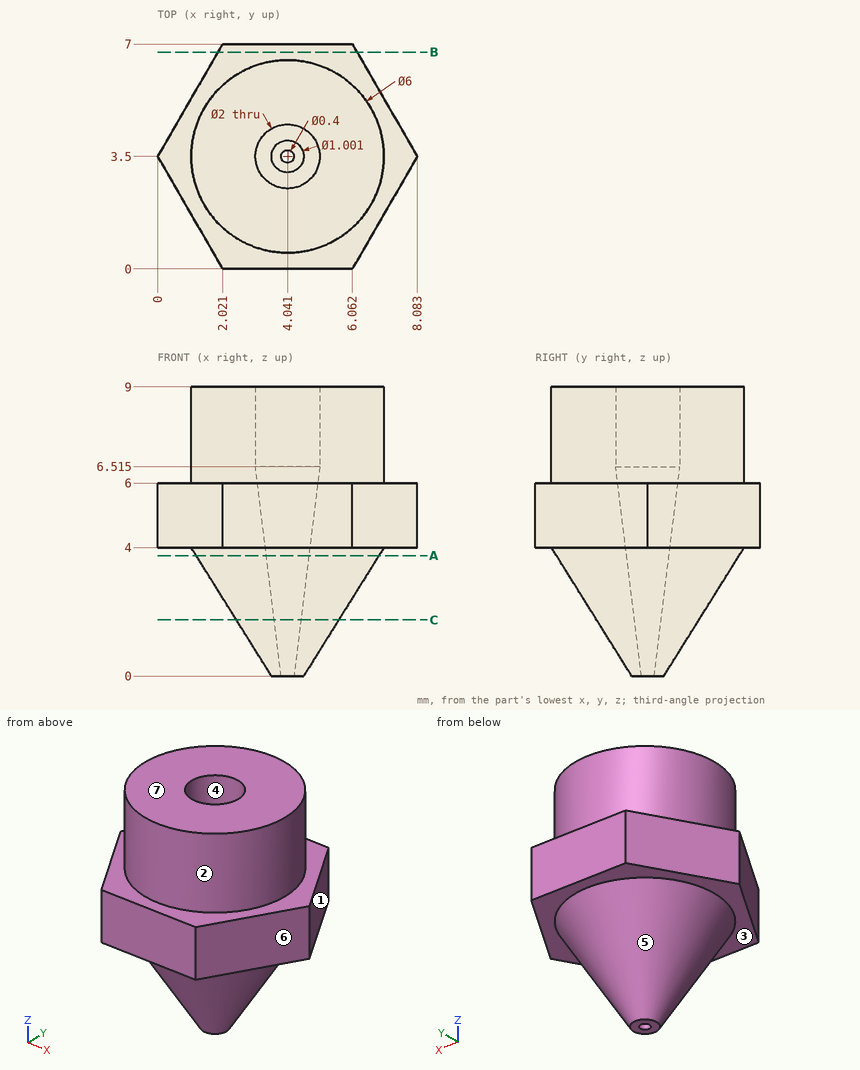
Verification items for this drawing (mm, ordinates from the low corner). A direction names the side the tool comes from. Coordinates: 2 decimals unless noted, no trailing zeros. Write each loop counter-clockwise with the first axis right and the second up, starting at its lowest first coordinate (ties: lowest second). Pieces come first, ordered by that corner, then holes. Notation, with made-up numbers: M 64,45 L 92,45 A25 cw 92,82 Z; hole C 89,78 d8. An arc over 180 degrees is marked long. Use CSV: the item, a comma, the result in double quotes.
Q1. Section check B-B, the plane y = 6.75. Enter the section's corners in (x, z).
Computed values:
outline,"M 1.88,4 L 6.21,4 L 6.21,6 L 1.88,6 Z"
Q2. Section check C-C, the plane z = 1.75. Enter the section's corners in (x, y) (1 decimal).
Computed values:
outline,"C 4,3.5 d3.2; hole C 4,3.5 d0.8"
Q3. Go/stop test with flat-tipped pins: P1, Ø2, axis at x = 6.5, z = 8, coming from the -Y side; P2, Ø2, axis at x = 6, y = 4.5, coming from the -Z side; P3, Ø4, axis at x = 6.5, y = 6, coming from the -Z side. Record where each tip stops, or that it passes through.
Computed values:
P1,"y = 0.88"
P2,"z = 1.12"
P3,"z = 1.61"
Q4. Thickness scan on line 1 along Y through (x, z) = (4, 1.5); line 2 along Z through (x, y) = (2.25, 5.5) (1 decimal); line 3 along Z through (x, y) = (7.5, 4). Record the ranges inside material, lowest first. Write a range as [from, to].
Computed values:
line 1,"[2.06, 3.12], [3.88, 4.94]"
line 2,"[3.5, 9]"
line 3,"[4, 6]"
Q5. Set-up check for the marked faces 1, 2 and 3: record each of +Z, -Z, +X, -X, +Y, -Y from which the full face is reachable in a straight line by a thin tool's end or side.
Computed values:
face 1,"+Z, -Z, +X, +Y"
face 2,"+Z"
face 3,"-Z"
Q6. Section check A-A, the plane z = 3.75. Enter the section's corners in (x, y) (1 decimal).
Computed values:
outline,"C 4,3.5 d5.7; hole C 4,3.5 d1.3"
Q7. Mould release check, pull along Y, two halves, no side actions. Record for the marked faces 4, 5, 6 and 7: pulls with the +Y half, pulls with the -Y half, needs draft (parallel to the pull), parting line crosses it, or undercut.
Computed values:
face 4,"undercut"
face 5,"parting line crosses it"
face 6,"pulls with the -Y half"
face 7,"needs draft"
